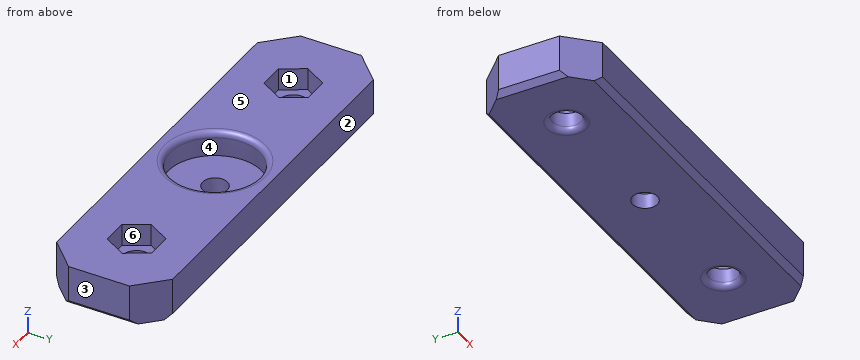
from build123d import *

# Parameters (mm, degrees)
SKETCH1_W           = 74
SKETCH1_H           = 21
BOSS_EXTRUDE1_DEPTH = 7.5
SKETCH2_R           = 8
CUT_EXTRUDE1_DEPTH  = 4.75
CUT_EXTRUDE1_TAPER  = -6
SKETCH4_R           = 2.6
CUT_EXTRUDE4_DEPTH  = 8.5000001
CHAMFER3_SIZE       = 5
CUT_EXTRUDE6_DEPTH  = 4
SKETCH11_R          = 2.25
CUT_EXTRUDE10_DEPTH = 8.5
FILLET4_R           = 1
FILLET5_R           = 1
CHAMFER5_SIZE       = 1


with BuildPart() as part:
    # Sketch1 → Boss-Extrude1 (new body)
    with BuildSketch(Plane.XY):
        Rectangle(SKETCH1_W, SKETCH1_H)
    extrude(amount=BOSS_EXTRUDE1_DEPTH)

    # Sketch2 → Cut-Extrude1 (cut)
    with BuildSketch(Plane.XY.offset(7.5)):
        Circle(SKETCH2_R)
    extrude(amount=-CUT_EXTRUDE1_DEPTH, taper=CUT_EXTRUDE1_TAPER, mode=Mode.SUBTRACT)

    # Sketch4 → Cut-Extrude4 (cut, through all)
    with BuildSketch(Plane(origin=(0, 0, 0), x_dir=(-1, 0, 0), z_dir=(0, 0, -1))):
        with Locations((-25, 0)):
            Circle(SKETCH4_R)
        with Locations((25, 0)):
            Circle(SKETCH4_R)
    extrude(amount=-CUT_EXTRUDE4_DEPTH, mode=Mode.SUBTRACT)

    # Chamfer3
    chamfer3_edges = [part.edges().sort_by_distance(p)[0] for p in [
        (37, -10.5, 3.75),
        (-37, -10.5, 3.75),
        (-37, 10.5, 3.75),
        (37, 10.5, 3.75),
    ]]
    chamfer(chamfer3_edges, length=CHAMFER3_SIZE)

    # Sketch5 → Cut-Extrude6 (cut)
    with BuildSketch(Plane.XY.offset(7.5)):
        Polygon((22.690598923, -4), (27.309401077, -4), (29.618802154, 0), (27.309401077, 4), (22.690598923, 4), (20.381197846, 0), align=None)
        Polygon((-27.309401077, -4), (-22.690598923, -4), (-20.381197846, 0), (-22.690598923, 4), (-27.309401077, 4), (-29.618802154, 0), align=None)
    extrude(amount=-CUT_EXTRUDE6_DEPTH, mode=Mode.SUBTRACT)

    # Sketch11 → Cut-Extrude10 (cut, through all)
    with BuildSketch(Plane.XY.offset(7.5)):
        Circle(SKETCH11_R)
    extrude(amount=-CUT_EXTRUDE10_DEPTH, mode=Mode.SUBTRACT)

    # Fillet4
    fillet4_edges = [part.edges().sort_by_distance(p)[0] for p in [
        (27.6, 0, 0),
        (-22.4, 0, 0),
    ]]
    fillet(fillet4_edges, radius=FILLET4_R)

    # Fillet5
    fillet5_edges = [part.edges().sort_by_distance(p)[0] for p in [
        (-8, 0, 7.5),
    ]]
    fillet(fillet5_edges, radius=FILLET5_R)

    # Chamfer5
    chamfer5_edges = [part.edges().sort_by_distance(p)[0] for p in [
        (-37, 0, 0),
        (37, 0, 0),
        (0, -10.5, 0),
        (0, 10.5, 0),
    ]]
    chamfer(chamfer5_edges, length=CHAMFER5_SIZE)


solid = part.part
Here's how the part is built. I have some questions about the finished solid (model axes, mm). Face numbers are marked on the shaded views. A direction names the side the tool comes from. Give positions to 0.01 mm unless a question says otherwise; leave off trailing zeros. Order: outer loops, then holes, each group sorted by start corner. A loop starts at its lowest first (then second) coordinate and runs counter-clockwise, first axis right, second up. Notation, with made-up numbers: (-14.5, 83.5) -> (16.5, 83.5) arc R16 ccw to (16.5, 112.5) -> close; hole circle Ø1 at (-21, -9). An arc over 180 degrees is marked (long way). Use a Markdown table: item, result. Add a question column.
Item 1: Imagine slicing it at D-D on y = 1. Give the number of separate pieces and of enclosed holes in the cut face, plus the area to 3 significant figures.
Item 2: If we mould it in two halves opening along Y, with no side actions, what happens to the marked faces 1, 2 and 3? For each: pulls with the +Y half, pulls with the -Y half, needs draft (parallel to the pull), parting line crosses it, or undercut.
Item 3: I need wall thicknesses on line 1 (Z direction, x = -6, y = -1.5); line 2 (Y direction, x = -25, z = 2.4); line 3 (X direction, y = -1, z = 6.75). Which ranges of each line are inside material? Lowest first, please.
Item 4: For the marked faces 4, 5 and 6, which set-ups out of +Z, -Z, +X, -X, +Y, -Y let a thin tool reach every point of the face, with its end or its side?
Item 5: Will these pins go through, and if not, where does the flat tip stop? pin 1 (5 mm diameter, centred on x = 0, y = 0, fed in from -Z); pin 2 (5 mm diameter, centred on x = 0, y = 2.5, fed in from +Z); pin 3 (2.5 mm diameter, centred on x = 25, y = -1.5, fed in from +Z).
Item 6: Imagine slicing it at C-C on x = 0. Please give me the cut outline in (y, z), plus the area to 3 significant figures.
Item 7: Imagine slicing it at A-A on x = 25. Please give me the cut outline in (y, z).
Item 8: Imagine slicing it at B-B on z = 5.5. Please give me the cut outline in (x, y).
Data:
| question | item | result |
|---|---|---|
| 1 | separate pieces | 4 |
| 1 | enclosed holes | 0 |
| 1 | area | 365 mm² |
| 2 | face 1 | undercut |
| 2 | face 2 | pulls with the +Y half |
| 2 | face 3 | needs draft |
| 3 | line 1 | z = 0 to 2.75 |
| 3 | line 2 | y = -10.5 to -2.6, 2.6 to 10.5 |
| 3 | line 3 | x = -37 to -29.04, -20.96 to -8.08, 8.08 to 20.96, 29.04 to 37 |
| 4 | face 4 | none |
| 4 | face 5 | +Z, +X, -X, +Y, -Y |
| 4 | face 6 | +Z |
| 5 | pin 1 | stops at z = 0 |
| 5 | pin 2 | stops at z = 2.75 |
| 5 | pin 3 | stops at z = 3.5 |
| 6 | outline | (-10.5, 1) -> (-9.5, 0) -> (-2.25, 0) -> (-2.25, 2.75) -> (-8.5, 2.75) -> (-8.12, 6.4) arc R1 ccw to (-9.11, 7.5) -> (-10.5, 7.5) -> close; (2.25, 0) -> (9.5, 0) -> (10.5, 1) -> (10.5, 7.5) -> (9.11, 7.5) arc R1 ccw to (8.12, 6.4) -> (8.5, 2.75) -> (2.25, 2.75) -> close |
| 6 | area | 65.2 mm² |
| 7 | outline | (-10.5, 1) -> (-9.5, 0) -> (-3.6, 0) arc R1 ccw to (-2.6, 1) -> (-2.6, 3.5) -> (-4, 3.5) -> (-4, 7.5) -> (-10.5, 7.5) -> close; (2.6, 1) arc R1 ccw to (3.6, 0) -> (9.5, 0) -> (10.5, 1) -> (10.5, 7.5) -> (4, 7.5) -> (4, 3.5) -> (2.6, 3.5) -> close |
| 8 | outline | (-37, -5.5) -> (-32, -10.5) -> (32, -10.5) -> (37, -5.5) -> (37, 5.5) -> (32, 10.5) -> (-32, 10.5) -> (-37, 5.5) -> close; hole (-29.62, 0) -> (-27.31, -4) -> (-22.69, -4) -> (-20.38, 0) -> (-22.69, 4) -> (-27.31, 4) -> close; hole circle Ø16.42 at (0, 0); hole (20.38, 0) -> (22.69, -4) -> (27.31, -4) -> (29.62, 0) -> (27.31, 4) -> (22.69, 4) -> close |
